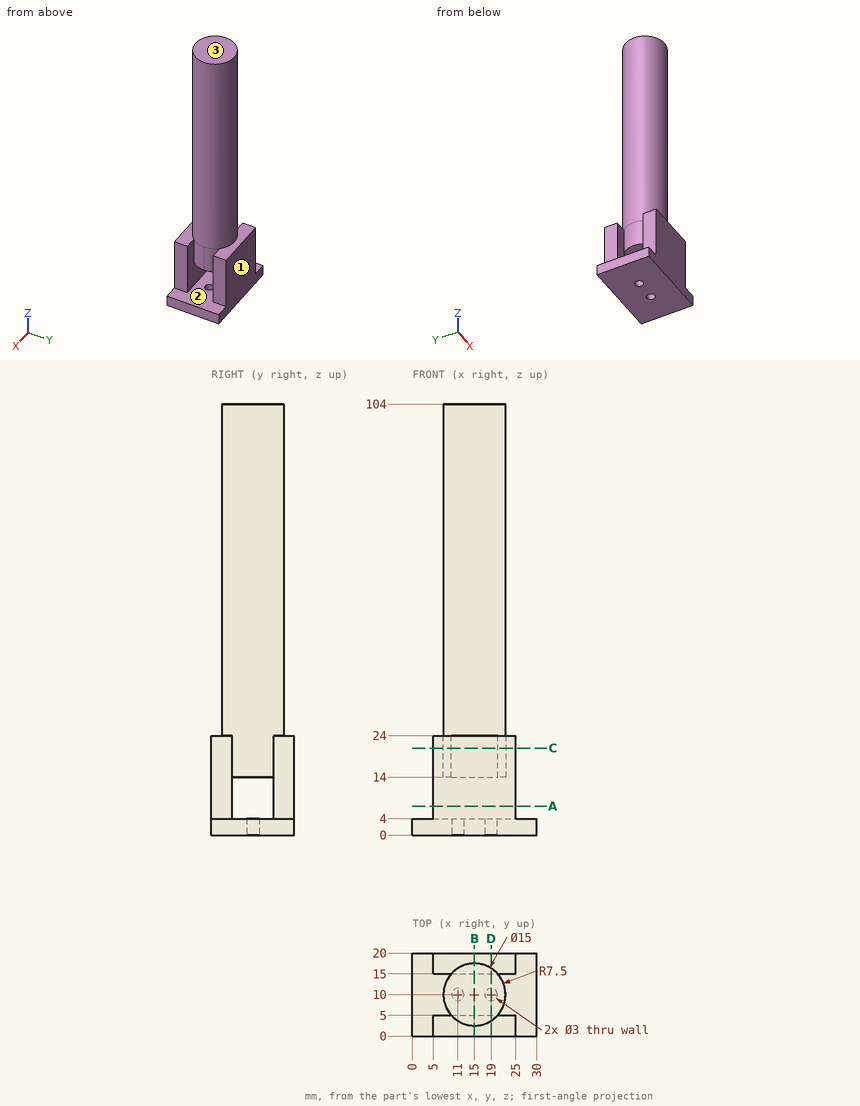
Part print with two shaded views. Sizes in mm from the minimum x, y, z corner. Give positions to 0.01 mm unless a question says otherwise; leave off trailing zeros. Order: outer loops, then holes, each group sorted by start corner. A loop starts at its lowest first (then second) coordinate and runs counter-clockwise, first axis right, second up. Notation, with made-up numbers: M -7,29.25 L 17,29.25 A17 ccw 17,55.25 Z; hole C 89,-23.75 d10. An arc over 180 degrees is marked long. Use one line per item in the form item = value.
1) Saw through at B-B (x = 15). Give the cut face in (y, z), plus the area to 3 significant figures.
Calculated:
outline = M 0,0 L 20,0 L 20,24 L 17.5,24 L 17.5,104 L 2.5,104 L 2.5,24 L 0,24 Z; hole M 5,4 L 15,4 L 15,14 L 5,14 Z
area = 1,580 mm2
2) Saw through at C-C (z = 21). Give the cut face in (x, y), plus the area to 3 significant figures.
Calculated:
outline = M 5,0 L 25,0 L 25,5 L 20.59,5 A7.5 ccw 20.59,15 L 25,15 L 25,20 L 5,20 L 5,15 L 9.41,15 A7.5 ccw 9.41,5 L 5,5 Z
area = 338 mm2
3) Saw through at D-D (x = 19). Give the cut face in (y, z).
Calculated:
outline = M 0,0 L 8.5,0 L 8.5,4 L 5,4 L 5,14 L 15,14 L 15,4 L 11.5,4 L 11.5,0 L 20,0 L 20,24 L 16.34,24 L 16.34,104 L 3.66,104 L 3.66,24 L 0,24 Z
4) Saw through at A-A (z = 7). Give the cut face in (x, y).
Calculated:
outline = M 5,0 L 25,0 L 25,5 L 5,5 Z; M 5,15 L 25,15 L 25,20 L 5,20 Z
5) Drop flat-ended pins along their axis: pin 1 (5.5 mm diameter, centred on y = 17.5, z = 14, fed in from -X); pin 2 (5.5 mm diameter, centred on y = 17, z = 11, fed in from +X); pin 3 (6 mm diameter, centred on x = 4, z = 86, fed in from +Y); pin 4 (2 mm diameter, centred on y = 4.5, z = 58, fed in from -X). Give the stop position or say it passes through.
Calculated:
pin_1 = 5
pin_2 = 25
pin_3 = through
pin_4 = 9
6) Two-plate mould, pull along Z, no slides. Class the marked faces 1, 2 and 3: released by +Z, released by -Z, zero draft, split by the parting line, or undercut.
Calculated:
face_1 = zero draft
face_2 = undercut
face_3 = released by +Z
7) Probe probe 1 along Y at (x, z) = (19, 1.5); probe 2 along Z at (x, y) = (9.75, 12.5); probe 3 along Y at (x, z) = (5.75, 17.5). List the from-to ranges inside material, lowest first.
Calculated:
probe_1 = 0 to 8.5, 11.5 to 20
probe_2 = 0 to 4, 14 to 104
probe_3 = 0 to 5, 15 to 20
